Input: dimensioned drawing with shaded views. Units: mm. Origin: part minimum x, y, z. A direction names the side the tool comes from. Coordinates: 2 decimals unless noted, no trailing zeros. Loops run counter-clockwise (first coordinate to the right, second up) from the corner with the lowest first, then second, coordinate; pieces in that order, holes last.
(1) Contact query for flat-ended pins moving along their axis: P1, Ø3, axis at y = 1.5, z = 3.5, coming from the +X side; P2, Ø3.5, axis at x = 30.93, y = 4, coming from the -Z side; P3, Ø2, axis at x = 20.5, z = 13.5, coming from the +Y side. Output: stop coordinate, or through.
(2) Line query: L1, parallel to X at y = 2.75, z = 14.5 (1 decimal); L2, parallel to X at y = 1.5, z = 12.75 (1 decimal); L3, parallel to X at y = 5.75, z = 12.25 (1 decimal). Output: solid intervals per line, ascending.
(3) Section B-B, the plane x = 4. Return loops of the section in (y, z) (1 decimal).
(4) Section D-D, the plane y = 6. Return loops of the section in (x, z) (1 decimal).
(5) Section C-C, the plane z = 8.25. Return loops of the section in (x, y) (1 decimal).
(6) Set-up query: the marked faces 5 and 6. Return all of +Z, -Z, +X, -X, +Y, -Y with unobstructed straight access to the full face (end or side cutting, diameter ignored); none if empty.
(7) Section A-A, the plane y = 4. Return loops of the section in (x, z) (1 decimal).
(8) Mould query, pull axis Y, two halves, no side actions, for the marked faces 1, 2, 3 and 4. Classes: released by +Y, released by -Y, zero draft, split by the parting line, or undercut.
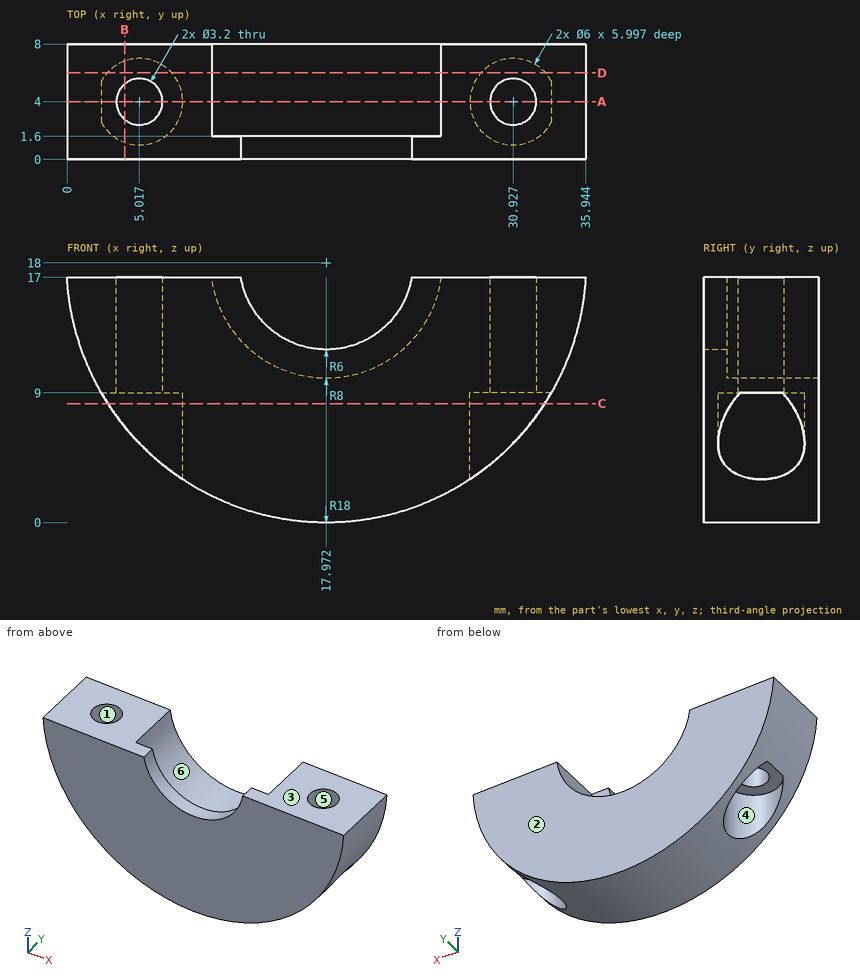
Report:
1. P1: stops at x = 30.35
1. P2: stops at z = 9
1. P3: stops at y = 1.6
2. L1: x = 0.3 to 4, 6 to 10.8, 25.2 to 29.9, 31.9 to 35.6
2. L2: x = 0.8 to 15.1, 20.9 to 35.2
2. L3: x = 0.9 to 12.4, 23.5 to 35
3. outline: (0, 6.7) - (1.2, 6.7) - (1.2, 9) - (2.8, 9) - (2.8, 17) - (0, 17) - close; (5.2, 9) - (6.8, 9) - (6.8, 6.7) - (8, 6.7) - (8, 17) - (5.2, 17) - close
4. outline: (0, 17) arc R18 ccw to (2.8, 8.3) - (2.8, 9) - (7.3, 9) - (7.3, 3.5) arc R18 ccw to (28.7, 3.5) - (28.7, 9) - (33.2, 9) - (33.2, 8.3) arc R18 ccw to (35.9, 17) - (25.9, 17) arc R8 cw to (10, 17) - close
5. outline: (2.8, 0) - (33.1, 0) - (33.1, 1.9) arc R3 cw (long way) to (33.1, 6.1) - (33.1, 8) - (2.8, 8) - (2.8, 6.1) arc R3 cw (long way) to (2.8, 1.9) - close
6. face 5: +Z, -Z
6. face 6: +Z, +Y
7. outline: (0, 17) arc R18 ccw to (2.4, 9) - (3.4, 9) - (3.4, 17) - close; (6.6, 9) - (8, 9) - (8, 3) arc R18 ccw to (27.9, 3) - (27.9, 9) - (29.3, 9) - (29.3, 17) - (25.9, 17) arc R8 cw to (10, 17) - (6.6, 17) - close; (32.5, 9) - (33.6, 9) arc R18 ccw to (35.9, 17) - (32.5, 17) - close
8. face 1: undercut
8. face 2: released by +Y
8. face 3: zero draft
8. face 4: undercut
